from build123d import *

# Parameters (mm, degrees)
F0_R     = 11
F1_DEPTH = 7


with BuildPart() as f1:
    # F0 (on Right) → F1 (new body)
    with BuildSketch(Plane.YZ):
        with BuildLine():
            ThreePointArc((-10.784147298, -2.158380433), (-15.2181462376, 1.0504484301), (-20.5081756924, 2.4549118995))
            ThreePointArc((-20.5081756924, 2.4549118995), (-21.7006480739, 2.3804655364), (-22.893620827, 2.4464098455))
            ThreePointArc((-22.893620827, 2.4464098455), (-33.994808864, -21.019176627), (-8.1163913394, -18.9752512981))
            ThreePointArc((-8.1163913394, -18.9752512981), (-7.0194101473, -15.8207684356), (-6.6476058185, -12.5017487903))
            ThreePointArc((-6.6476058185, -12.5017487903), (-6.8012263567, -10.3604835388), (-7.2589414021, -8.2630772634))
            ThreePointArc((-7.2589414021, -8.2630772634), (-9.5238156568, -5.500769422), (-10.784147298, -2.158380433))
        make_face()
        with Locations((-21.6476058185, -12.5017487903)):
            Circle(F0_R, mode=Mode.SUBTRACT)
        with BuildLine():
            ThreePointArc((-3.5235349877, 10.4197153255), (-8.5198228728, 12.6544494568), (-12.381765286, 16.532893741))
            ThreePointArc((-12.381765286, 16.532893741), (-12.9305392328, 7.4652234928), (-20.5081756924, 2.4549118995))
            ThreePointArc((-20.5081756924, 2.4549118995), (-15.2181462376, 1.0504484301), (-10.784147298, -2.158380433))
            ThreePointArc((-10.784147298, -2.158380433), (-9.5247042237, 5.4992305421), (-3.5235349877, 10.4197153255))
        make_face()
        with BuildLine():
            ThreePointArc((12.3770934621, 16.5260660004), (14.3292777545, 20.564709814), (15, 25))
            ThreePointArc((15, 25), (-3.2778125884, 39.6374842318), (-13.5674592847, 18.602809323))
            ThreePointArc((-13.5674592847, 18.602809323), (-12.9137018843, 17.6027423738), (-12.381765286, 16.532893741))
            ThreePointArc((-12.381765286, 16.532893741), (-8.5198228728, 12.6544494568), (-3.5235349877, 10.4197153255))
            ThreePointArc((-3.5235349877, 10.4197153255), (0.0011309034, 11.0000000457), (3.5258904978, 10.4202847697))
            ThreePointArc((3.5258904978, 10.4202847697), (8.5174154423, 12.6527884045), (12.3770934621, 16.5260660004))
        make_face()
        with Locations((-0.0030291348, 24.9982509651)):
            Circle(F0_R, mode=Mode.SUBTRACT)
        with BuildLine():
            ThreePointArc((20.5011537716, 2.457407484), (12.9303431289, 7.4655631547), (12.3770934621, 16.5260660004))
            ThreePointArc((12.3770934621, 16.5260660004), (8.5174154423, 12.6527884045), (3.5258904978, 10.4202847697))
            ThreePointArc((3.5258904978, 10.4202847697), (8.9396528624, 6.4123872618), (11.0020194703, 8.16e-08))
            ThreePointArc((11.0020194703, 8.16e-08), (10.9485181944, -1.0835891777), (10.7885348007, -2.1566378173))
            ThreePointArc((10.7885348007, -2.1566378173), (15.2171845533, 1.0506135401), (20.5011537716, 2.457407484))
        make_face()
        with BuildLine():
            ThreePointArc((36.6536642295, -12.4982509651), (31.8446490477, -1.4917152506), (20.5011537716, 2.457407484))
            ThreePointArc((20.5011537716, 2.457407484), (15.2171845533, 1.0506135401), (10.7885348007, -2.1566378173))
            ThreePointArc((10.7885348007, -2.1566378173), (9.5287431643, -5.4992303789), (7.2643152111, -8.261904092))
            ThreePointArc((7.2643152111, -8.261904092), (6.7026707945, -13.7097769898), (8.1341442138, -18.9961412801))
            ThreePointArc((8.1341442138, -18.9961412801), (8.7894001381, -19.9846100473), (9.3251094568, -21.0426489671))
            ThreePointArc((9.3251094568, -21.0426489671), (26.1298053359, -26.8148204143), (36.6536642295, -12.4982509651))
        make_face()
        with Locations((21.6506349533, -12.4965021748)):
            Circle(F0_R, mode=Mode.SUBTRACT)
        with BuildLine():
            ThreePointArc((8.1341442138, -18.9961412801), (6.7026707945, -13.7097769898), (7.2643152111, -8.261904092))
            ThreePointArc((7.2643152111, -8.261904092), (0.0029080373, -10.9999998825), (-7.2589414021, -8.2630772634))
            ThreePointArc((-7.2589414021, -8.2630772634), (-6.8012263567, -10.3604835388), (-6.6476058185, -12.5017487903))
            ThreePointArc((-6.6476058185, -12.5017487903), (-7.0194101473, -15.8207684356), (-8.1163913394, -18.9752512981))
            ThreePointArc((-8.1163913394, -18.9752512981), (0.0140889918, -14.9307955749), (8.1341442138, -18.9961412801))
        make_face()
    extrude(amount=F1_DEPTH)


solid = f1.part
Model file for the job. Use its own axes, mm. Coordinates: 2 decimals unless noted, no trailing zeros. Loops run counter-clockwise (first coordinate to the right, second up) from the corner with the lowest first, then second, coordinate; pieces in that order, holes last. Notation, with made-up numbers: (-33, -14.75) -> (-15, -14.75) arc R26 cw to (-15, 14.25) -> close; hole circle Ø6 at (44.25, 23). An arc over 180 degrees is marked (long way). Use one line per item in the form item = value. Start each with the question number.
(1) Pull direction Z, two halves, no side cores. Call faces 1 (the cylindrical face through (3.45, 13, 7.35)), 2 (the cylindrical face through (3.45, 1.63, 39.91)), 3 (the cylindrical face through (3.45, -34.24, -20.65)), 4 (the flat face through (7, 3, -11)): pulls with the +Z half, pulls with the -Z half, needs draft (parallel to the pull), parting line crosses it, or undercut.
(2) Cut at C-C on x = 3. Give the cut face in (y, z).
(3) Flat gauge pins, fed straight in: pin 1 (2 mm diameter, centred on x = 5.5, y = 0, fed in from -Z); pin 2 (13 mm diameter, centred on y = -21.65, z = -12.5, fed in from +X); pin 3 (4 mm diameter, centred on x = 2, y = -1, fed in from -Z). Where does each tip first touch, or does it go through?
(4) Probe probe 1 along Y at (x, z) = (1.75, -12); probe 2 along Z at (x, y) = (3.5, 0.5); probe 3 along Z at (x, y) = (5.25, 2). List the from-to ranges inside material, lowest first. Write a range as from..to.
(5) Cut at A-A on y = 0. Give the cut face in (x, z).
(6) Cut at B-B on z = -17.5. Give the cut face in (x, y), and give its area (3 significant figures).
Values:
q1.face_1 = undercut
q1.face_2 = undercut
q1.face_3 = parting line crosses it
q1.face_4 = needs draft
q2.outline = (-22.89, 2.45) arc R15 ccw (long way) to (-8.12, -18.98) arc R10.17 cw to (9.33, -21.04) arc R15 ccw (long way) to (20.5, 2.46) arc R10.17 cw to (12.38, 16.53) arc R15 ccw (long way) to (-13.57, 18.6) arc R10.17 cw to start; hole circle Ø22 at (-21.65, -12.5); hole circle Ø22 at (0, 0); hole circle Ø22 at (0, 25); hole circle Ø22 at (21.65, -12.5)
q3.pin_1 = -14.98
q3.pin_2 = through
q3.pin_3 = -15.38
q4.probe_1 = -36.64..-32.64, -10.66..10.66, 32.64..36.65
q4.probe_2 = -14.94..-10.99, 10.99..14.01, 35.99..39.99
q4.probe_3 = -15.13..-10.82, 10.82..14.18, 35.81..39.87
q5.outline = (0, -14.93) -> (7, -14.93) -> (7, -11) -> (0, -11) -> close; (0, 11) -> (7, 11) -> (7, 14) -> (0, 14) -> close; (0, 36) -> (7, 36) -> (7, 40) -> (0, 40) -> close
q6.outline = (0, -35.79) -> (7, -35.79) -> (7, -31.45) -> (0, -31.45) -> close; (0, -11.85) -> (7, -11.85) -> (7, -6.76) -> (0, -6.76) -> close; (0, 6.76) -> (7, 6.76) -> (7, 11.85) -> (0, 11.85) -> close; (0, 31.45) -> (7, 31.45) -> (7, 35.8) -> (0, 35.8) -> close
q6.area = 132 mm2
